from build123d import *

# Parameters (mm, degrees)
F1_DEPTH = 1
F2_W     = 1
F2_H     = 90
F3_DEPTH = 10


with BuildPart() as f1:
    # F0 (on Front) → F1 (new body)
    with BuildSketch(Plane.XZ):
        Polygon((111, -49.083949), (111, 40.916051), (60.5, 40.916051), (0, 40.916051), (-111, 40.916051), (-111, -49.083949), align=None)
    extrude(amount=F1_DEPTH)

    # F2 (on face) → F3 (join)
    with BuildSketch(Plane(origin=(0, 0, 0), x_dir=(-1, 0, 0), z_dir=(0, 1, 0))):
        with Locations((-110.5, -4.083949)):
            Rectangle(F2_W, F2_H)
        with Locations((110.5, -4.083949)):
            Rectangle(F2_W, F2_H)
    extrude(amount=F3_DEPTH)


solid = f1.part
Here's how the part is built. I have some questions about the finished solid (model axes, mm). A direction names the side the tool comes from. Coordinates: 2 decimals unless noted, no trailing zeros. Order: outer loops, then holes, each group sorted by start corner. A loop starts at its lowest first (then second) coordinate and runs counter-clockwise, first axis right, second up.
Item 1: For faces 1 (the face through (0.5, -0.4, 40.916)), 2 (the face through (-2, 0, -3)), which set-ups out of +Z, -Z, +X, -X, +Y, -Y let a thin tool reach every point of the face, with its end or its side?
Result sheet:
face 1: +Z, +X, -X, +Y, -Y
face 2: +Z, -Z, +Y
Item 2: For P1, Ø5, axis at x = 87, y = 4, coming from the +Z side; P2, Ø2, axis at x = 20.5, z = 10, coming from the +Y side, each with a flat end and sliding along its axis, tell me the tip position at first contact or that it passes through.
Result sheet:
P1: passes through
P2: stops at y = 0
Item 3: If we section it at B-B on z = 35.5: List the corners of the cut face in (x, y) for me.
Result sheet:
outline: (-111, -1) - (111, -1) - (111, 10) - (110, 10) - (110, 0) - (-110, 0) - (-110, 10) - (-111, 10) - close
Item 4: I need wall thicknesses on line 1 (X direction, y = 4.5, z = -11.5); line 2 (Y direction, x = -32.5, z = -16.5). Which ranges of each line are inside material? Lowest first, please.
Result sheet:
line 1: x = -111 to -110, 110 to 111
line 2: y = -1 to 0
Item 5: If we section it at A-A on y = 3: List the corners of the cut face in (x, z) for me.
Result sheet:
outline: (-111, -49.08) - (-110, -49.08) - (-110, 40.92) - (-111, 40.92) - close; (110, -49.08) - (111, -49.08) - (111, 40.92) - (110, 40.92) - close
Item 6: If we section it at C-C on x = -43: List the corners of the cut face in (y, z) for me.
Result sheet:
outline: (-1, -49.08) - (0, -49.08) - (0, 40.92) - (-1, 40.92) - close
Item 7: If we mould it in two halves opening along X, with no side actions, what happens to faces 3 (the face through (110, 5, -5)), 4 (the face through (-111, 5, -3)), 5 (the face through (0.5, -0.4, -49.084))? For each: +X half, -X half, draft (parallel to the pull), parting line (faces both ways), or undercut.
Result sheet:
face 3: undercut
face 4: -X half
face 5: draft
